Work out the finished part from the listing and answer in its coordinate system (mm). Face numbers are marked on the shaded views. A direction names the side the tool comes from. Give positions to 0.01 mm unless a question says otherwise; leave off trailing zeros. Order: outer loops, then holes, each group sorted by start corner. A loop starts at its lowest first (then second) coordinate and runs counter-clockwise, first axis right, second up. Notation, with made-up numbers: (61.25, 15.5) - (80.25, 15.5) arc R33 ccw to (80.25, 53.5) - close; hole circle Ø10 at (77.25, 64.25). An arc over 180 degrees is marked (long way). Put each result on its own line as item: value.
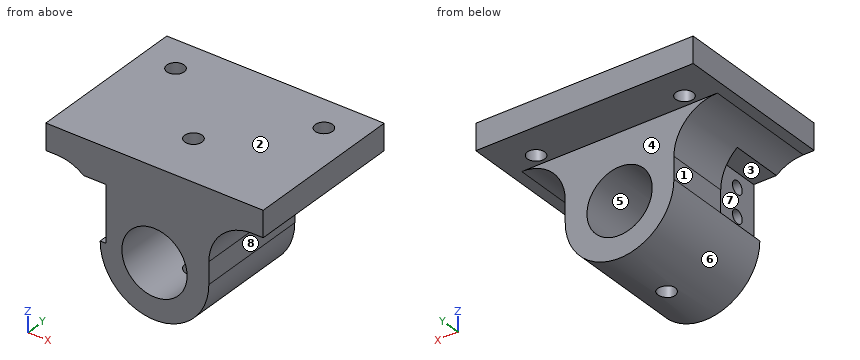
```python
from build123d import *

# Parameters (mm, degrees)
PROFILE_SKETCH1_R                          = 7.5
PROFILE_BOSS_EXTRUDE2_DEPTH                = 37.25987
FASTENINGHOLESKETCH3_R                     = 2
FASTENINGHOLECUT_EXTRUDE8_DEPTH            = 56.995963358
LM8UUFASTENINGHOLESKETCH5_R                = 2
LM8UUFASTENINGHOLECUT_EXTRUDE9_DEPTH       = 56.995963425
TOPKNOTCHSKETCH2_W                         = 50
TOPKNOTCHSKETCH2_H                         = 27.5
TOPKNOTCHCUT_EXTRUDE1_DEPTH                = 10.8
RIGHTZAXISMICROSWITCHCUT_EXTRUDE1_DEPTH    = 12.05
MICROSWITCHMOUNTINGHOLESSKETCH1_R          = 1.5
MICROSWITCHMOUNTINGHOLESCUT_EXTRUDE1_DEPTH = 3.1


with BuildPart() as part:
    # Profile-Sketch1 → Profile-Boss-Extrude2 (new body)
    with BuildSketch(Plane(origin=(0, 0, 0), x_dir=(1, 0, 0), z_dir=(0, 1, 0))):
        with BuildLine():
            Line((-25, -21), (25, -21))
            Line((25, -21), (25, -15))
            Line((25, -15), (22.5, -15))
            ThreePointArc((22.5, -15), (15.428932188, -12.071067812), (12.5, -5))
            Line((12.5, -5), (12.5, 0))
            ThreePointArc((12.5, 0), (0, 12.5), (-12.5, 0))
            Line((-12.5, 0), (-12.5, -5))
            ThreePointArc((-12.5, -5), (-15.428932188, -12.071067812), (-22.5, -15))
            Line((-22.5, -15), (-25, -15))
            Line((-25, -15), (-25, -21))
        make_face()
        with Locations(Location((0, 0, 0), (0, 0, 270))):
            Circle(PROFILE_SKETCH1_R, mode=Mode.SUBTRACT)
    extrude(amount=PROFILE_BOSS_EXTRUDE2_DEPTH)

    # FasteningHoleSketch3 → FasteningHoleCut-Extrude8 (cut, through all)
    with BuildSketch(Plane.XY.offset(21)):
        with Locations((-17.0625, 29.32237)):
            Circle(FASTENINGHOLESKETCH3_R)
        with Locations((17.0625, 29.32237)):
            Circle(FASTENINGHOLESKETCH3_R)
    extrude(amount=-FASTENINGHOLECUT_EXTRUDE8_DEPTH, mode=Mode.SUBTRACT)

    # LM8UUFasteningHoleSketch5 → LM8UUFasteningHoleCut-Extrude9 (cut, through all)
    with BuildSketch(Plane.XY.offset(21)):
        with Locations((0, 12)):
            Circle(LM8UUFASTENINGHOLESKETCH5_R)
    extrude(amount=-LM8UUFASTENINGHOLECUT_EXTRUDE9_DEPTH, mode=Mode.SUBTRACT)

    # TopKnotchSketch2 → TopKnotchCut-Extrude1 (cut)
    with BuildSketch(Plane(origin=(0, 37.25987, 0), x_dir=(1, 0, 0), z_dir=(0, 1, 0))):
        with Locations((0, -1.25)):
            Rectangle(TOPKNOTCHSKETCH2_W, TOPKNOTCHSKETCH2_H)
    extrude(amount=-TOPKNOTCHCUT_EXTRUDE1_DEPTH, mode=Mode.SUBTRACT)

    # RightZAxisMicroSwitchSketch2 → RightZAxisMicroSwitchCut-Extrude1 (cut)
    with BuildSketch(Plane.XZ):
        Polygon((-11.1, 0), (-13.9, 0), (-13.9, 10.086005596), (-16.342618224, 12.85), (-13.9, 12.85), (-11.1, 12.85), align=None)
    extrude(amount=-RIGHTZAXISMICROSWITCHCUT_EXTRUDE1_DEPTH, mode=Mode.SUBTRACT)

    # MicroSwitchMountingHolesSketch1 → MicroSwitchMountingHolesCut-Extrude1 (cut)
    with BuildSketch(Plane.ZY.offset(11.1)):
        with Locations((3.25, 5.05)):
            Circle(MICROSWITCHMOUNTINGHOLESSKETCH1_R)
        with Locations((9.6, 5.05)):
            Circle(MICROSWITCHMOUNTINGHOLESSKETCH1_R)
    extrude(amount=-MICROSWITCHMOUNTINGHOLESCUT_EXTRUDE1_DEPTH, mode=Mode.SUBTRACT)


solid = part.part
```
(1) Section C-C, the plane x = -10 is taken. Write down the section's boundary in (y, z).
Geometry check:
outline: (0, -7.5) - (26.46, -7.5) - (26.46, 15) - (37.26, 15) - (37.26, 21) - (0, 21) - close; hole circle Ø3 at (5.05, 3.25); hole circle Ø3 at (5.05, 9.6)
(2) A tool of negligible diameter and unlimited length cuts with its end or side. For the marked faces 1, 2, 3 and 4, from which of +Z, -Z, +X, -X, +Y, -Y can it reach the whole face along a straight path? Write none if from no direction.
Geometry check:
face 1: -Z, -X, +Y, -Y
face 2: +Z, +X, -X, +Y, -Y
face 3: -X, -Y
face 4: -Z, +X, -X, +Y
(3) Straight lines are drawn through the part: line 1 (Y direction, x = 0, z = 13.75); line 2 (Y direction, x = -8.8, z = 3.25); line 3 (X direction, y = 13, z = 0). For each, find the intervals that lie inside material, in ascending order.
Geometry check:
line 1: y = 0 to 10, 14 to 26.46
line 2: y = 0 to 3.55, 6.55 to 26.46
line 3: x = -12.5 to -7.5, 7.5 to 12.5
(4) Section D-D, the plane z = 2.5 is taken. Write down the section's boundary in (x, y).
Geometry check:
outline: (-12.5, 12.05) - (-11.1, 12.05) - (-11.1, 6.35) - (-8, 6.35) - (-8, 3.75) - (-11.1, 3.75) - (-11.1, 0) - (-7.07, 0) - (-7.07, 26.46) - (-12.5, 26.46) - close; (7.07, 0) - (12.5, 0) - (12.5, 26.46) - (7.07, 26.46) - close
(5) Section B-B, the plane x = 0 is taken. Write down the section's boundary in (y, z).
Geometry check:
outline: (0, -12.5) - (10, -12.5) - (10, -7.5) - (0, -7.5) - close; (0, 7.5) - (10, 7.5) - (10, 21) - (0, 21) - close; (14, -12.5) - (26.46, -12.5) - (26.46, -7.5) - (14, -7.5) - close; (14, 7.5) - (26.46, 7.5) - (26.46, 15) - (37.26, 15) - (37.26, 21) - (14, 21) - close
(6) Section A-A, the plane y = 24 is taken. Write down the section's boundary in (x, z).
Geometry check:
outline: (-25, 15) - (-22.5, 15) arc R10 cw to (-12.5, 5) - (-12.5, 0) arc R12.5 ccw to (12.5, 0) - (12.5, 5) arc R10 cw to (22.5, 15) - (25, 15) - (25, 21) - (-25, 21) - close; hole circle Ø15 at (0, 0)
(7) Determine the mould class of the marked faces 5, 6, 7 and 8 for opening direction Z: pulls with the +Z half, pulls with the -Z half, needs draft (parallel to the pull), parting line crosses it, or undercut.
Geometry check:
face 5: undercut
face 6: pulls with the -Z half
face 7: undercut
face 8: needs draft
(8) Given pin 1 (10 mm diameter, centred on x = 13.5, y = 9.5, fed in from -Z); pin 2 (0.9 mm diameter, centred on y = 4.5, z = 9, fed in from -X); pin 3 (6 mm diameter, centred on y = 32, z = -5, fed in from -X); pin 4 (5.5 mm diameter, centred on y = 17.5, z = 3.5, fed in from +X), each flat-ended and moving along its own axis, determine where each tip first touches the part or whether it passes through.
Geometry check:
pin 1: stops at z = -9.17
pin 2: stops at x = -8
pin 3: passes through
pin 4: stops at x = 12.58
